from build123d import *

# Parameters (mm, degrees)
BOSS_EXTRUDE1_DEPTH = 5.588
FILLET1_R           = 2.794
BOSS_EXTRUDE2_DEPTH = 1.5875


with BuildPart() as part:
    # Sketch1 → Boss-Extrude1 (new body)
    with BuildSketch(Plane(origin=(0, 0, 0), x_dir=(1, 0, 0), z_dir=(0, 1, 0))):
        Polygon((0, 0), (7.14375, 0), (7.14375, 5.529702374), (38.772931664, 8.296897206), (38.285905374, 13.863633179), (7.14375, 11.139047626), (7.14375, 16.66875), (0, 16.66875), (0, 13.49375), (1.5875, 13.49375), (1.5875, 15.08125), (5.55625, 15.08125), (5.55625, 1.5875), (1.5875, 1.5875), (1.5875, 3.175), (0, 3.175), align=None)
    extrude(amount=BOSS_EXTRUDE1_DEPTH)

    # Fillet1
    fillet1_edges = [part.edges().sort_by_distance(p)[0] for p in [
        (22.958340832, 0, -6.91329979),
        (22.714827687, 0, -12.501340403),
        (22.958340832, 5.588, -6.91329979),
        (22.714827687, 5.588, -12.501340403),
    ]]
    fillet(fillet1_edges, radius=FILLET1_R - 0.0001)  # a hair under: the kernel refuses the full size

    # Sketch2 → Boss-Extrude2 (add)
    with BuildSketch(Plane(origin=(39.198778227, 0, -3.429448719), x_dir=(-0.08715574274766254, 0, -0.9961946980917452), z_dir=(0.9961946980917452, 0, -0.08715574274766254))):
        with BuildLine():
            Line((7.68004135, 5.588), (10.98204135, 5.588))
            Line((10.98204135, 5.588), (10.98204135, 0))
            Line((10.98204135, 0), (7.68004135, 0))
            ThreePointArc((7.68004135, 0), (4.88604135, 2.794), (7.68004135, 5.588))
        make_face()
    extrude(amount=-BOSS_EXTRUDE2_DEPTH)


solid = part.part
Here's how the part is built. I have some questions about the finished solid (model axes, mm). A direction names the side the tool comes from. Give positions to 0.01 mm unless a question says otherwise; leave off trailing zeros. Order: outer loops, then holes, each group sorted by start corner. A loop starts at its lowest first (then second) coordinate and runs counter-clockwise, first axis right, second up. Notation, with made-up numbers: (46.5, 54.5) -> (80.5, 54.5) arc R15 cw to (80.5, 81.5) -> close; hole circle Ø3 at (73, -39). An arc over 180 degrees is marked (long way). Use a Markdown table: item, result. Add a question column.
Item 1: If we mould it in two halves opening along Z, with no side actions, what happens to faces 1 (the face through (1, 3, -13.494)), 2 (the face through (0, 3, -2)), 3 (the face through (23.11, 0.84, -7.726))? For each: pulls with the +Z half, pulls with the -Z half, needs draft (parallel to the pull), parting line crosses it, or undercut.
Item 2: Imagine slicing it at C-C on y = 3.35. Please give me the cut outline in (x, z) (1 decimal).
Item 3: Imagine slicing it at B-B on y = 1.7. Please give me the cut outline in (x, z) (1 decimal).
Item 4: For faces 4 (the face through (4, 3, -16.669)), 5 (the face through (5.556, 3, -8)), 6 (the face through (37.46, 2.83, -14.3)), 7 (the face through (36.686, 3.014, -13.934)), 8 (the face through (23, 5, -8)), which set-ups out of +Z, -Z, +X, -X, +Y, -Y let a thin tool reach every point of the face, with its end or its side?
Item 5: I need wall thicknesses on line 1 (X direction, y = 2.85, z = -2.5); line 2 (Z direction, x = 5, y = 3.45); line 3 (X direction, y = 4, z = -4). Which ranges of each line are inside material? Lowest first, please.
Item 6: Will these pins go through, and if not, where does the flat tip stop? pin 1 (1.2 mm diameter, centred on x = 3, y = 4, fed in from +Z); pin 2 (3 mm diameter, centred on y = 3, z = -10, fed in from -X); pin 3 (1.7 mm diameter, centred on y = 3.5, z = -14, fed in from +X); pin 4 (3 mm diameter, centred on x = 28, z = -14, fed in from -Y).
Item 7: Imagine slicing it at A-A on z = -2.75. Please give me the cut outline in (x, y), plus the area to 3 significant figures.
Data:
| question | item | result |
|---|---|---|
| 1 | face 1 | undercut |
| 1 | face 2 | needs draft |
| 1 | face 3 | pulls with the +Z half |
| 2 | outline | (0, -16.7) -> (7.1, -16.7) -> (7.1, -11.1) -> (36.7, -13.7) -> (36.7, -14.2) -> (38.2, -14.4) -> (38.8, -8.4) -> (7.1, -5.6) -> (7.1, 0) -> (0, 0) -> (0, -3.2) -> (1.6, -3.2) -> (1.6, -1.6) -> (5.6, -1.6) -> (5.6, -15.1) -> (1.6, -15.1) -> (1.6, -13.5) -> (0, -13.5) -> close |
| 3 | outline | (0, -16.7) -> (7.1, -16.7) -> (7.1, -10.9) -> (36.7, -13.5) -> (36.7, -14.2) -> (38.2, -14.4) -> (38.8, -8.5) -> (7.1, -5.8) -> (7.1, 0) -> (0, 0) -> (0, -3.2) -> (1.6, -3.2) -> (1.6, -1.6) -> (5.6, -1.6) -> (5.6, -15.1) -> (1.6, -15.1) -> (1.6, -13.5) -> (0, -13.5) -> close |
| 4 | face 4 | -Z, +X, -X, +Y, -Y |
| 4 | face 5 | +Y, -Y |
| 4 | face 6 | -Z, +Y, -Y |
| 4 | face 7 | none |
| 4 | face 8 | +Z, +X, +Y |
| 5 | line 1 | x = 0 to 1.59, 5.56 to 7.14 |
| 5 | line 2 | z = -16.67 to -15.08, -1.59 to 0 |
| 5 | line 3 | x = 5.56 to 7.14 |
| 6 | pin 1 | stops at z = 0 |
| 6 | pin 2 | stops at x = 5.56 |
| 6 | pin 3 | stops at x = 38.35 |
| 6 | pin 4 | stops at y = 1.25 |
| 7 | outline | (0, 0) -> (1.59, 0) -> (1.59, 5.59) -> (0, 5.59) -> close; (5.56, 0) -> (7.14, 0) -> (7.14, 5.59) -> (5.56, 5.59) -> close |
| 7 | area | 17.7 mm² |
